Work out the finished part from the listing and answer in its coordinate system (mm). Face numbers are marked on the shaded views. A direction names the side the tool comes from. Round coordinates to 2 decimals unless told otherwise and drop trailing zeros. Order: outer loops, then holes, each group sorted by start corner. A loop starts at its lowest first (then second) coordinate and runs counter-clockwise, first axis right, second up. Notation, with made-up numbers: (39.5, -14.5) -> (93.5, -14.5) arc R30 cw to (93.5, 20.5) -> close; hole circle Ø6 at (-39.5, 13.25). An arc over 180 degrees is marked (long way). Use a Markdown table: item, result. Add a question column.
Item 1: For a pull along Y with two mould halves and no side action, classify the marked faces 1, 2 and 3 as +Y half, -Y half, draft (parallel to the pull), parting line (faces both ways), or undercut.
Item 2: A cutting plane is placed at C-C, the plane y = 49. Determine the outline of the cut face in (x, z), plus the area to 3 significant figures.
Item 3: A cutting plane is placed at B-B, the plane z = 6.25. Determine the outline of the cut face in (x, y).
Item 4: A tool of negligible diameter and unlimited length cuts with its end or side. For the marked faces 4 and 5, from which of +Z, -Z, +X, -X, +Y, -Y can it reach the whole face along a straight path? Write none if from no direction.
Item 5: A cutting plane is placed at A-A, the plane x = -25. Determine the outline of the cut face in (y, z).
Item 6: A cutting plane is placed at D-D, the plane y = -12. Determine the outline of the cut face in (x, z).
Item 7: Flat-ended cylindrical pins translate along their axes: P1, Ø3.5, axis at y = 11.5, z = 3, coming from the +X side; P2, Ø2, axis at x = 7, z = 4, coming from the -Y side; P3, Ø2, axis at x = 18.5, y = 28.5, coming from the +Z side; P4, Ø6, axis at x = 27.5, y = 39.5, coming from the +Z side. Find the tip coordinate at first contact, or state that the pin passes through.
Item 8: Find the intervals of material crossed by L1, parallel to Y at x = 7, z = 8.75; L2, parallel to Y at x = 26, z = 3.75; L3, parallel to Y at x = 25, z = 1.8, in increasing order. Write a range as [from, to].
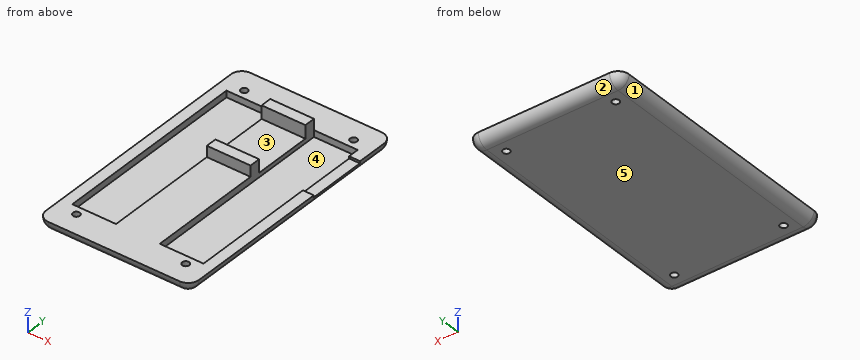
from build123d import *

# Parameters (mm, degrees)
SKETCH_1_W          = 70
SKETCH_1_H          = 118
EXTRUDE_1_DEPTH     = 40
SKETCH_2_W          = 64
SKETCH_2_H          = 112
CUT_EXTRUDE_1_DEPTH = 35
SKETCH_3_R          = 1.6
CUT_EXTRUDE_2_DEPTH = 78.012985918
FILLET_1_R          = 5
FILLET_2_R          = 5
SKETCH_4_W          = 80
SKETCH_4_H          = 120
CUT_EXTRUDE_3_DEPTH = 35
SKETCH_5_W          = 60
SKETCH_5_H          = 27
CUT_EXTRUDE_4_DEPTH = 1
SKETCH_6_W          = 20
SKETCH_6_H          = 90
CUT_EXTRUDE_5_DEPTH = 3
SKETCH_7_W          = 20
SKETCH_7_H          = 90
CUT_EXTRUDE_6_DEPTH = 3
SKETCH_8_W          = 20
SKETCH_8_H          = 5
EXTRUDE_2_DEPTH     = 5


with BuildPart() as part:
    # ｽｹｯﾁ1 → ﾎﾞｽ - 押し出し1 (new body)
    with BuildSketch(Plane.XY):
        Rectangle(SKETCH_1_W, SKETCH_1_H)
    extrude(amount=EXTRUDE_1_DEPTH)

    # ｽｹｯﾁ2 → ｶｯﾄ - 押し出し1 (cut)
    with BuildSketch(Plane.XY.offset(40)):
        Rectangle(SKETCH_2_W, SKETCH_2_H)
    extrude(amount=-CUT_EXTRUDE_1_DEPTH, mode=Mode.SUBTRACT)

    # ｽｹｯﾁ3 → ｶｯﾄ - 押し出し2 (cut, through all)
    with BuildSketch(Plane.XY.offset(5)):
        with Locations((-25, 49)):
            Circle(SKETCH_3_R)
        with Locations((25, 49)):
            Circle(SKETCH_3_R)
        with Locations((-25, -49)):
            Circle(SKETCH_3_R)
        with Locations((25, -49)):
            Circle(SKETCH_3_R)
    extrude(amount=-CUT_EXTRUDE_2_DEPTH, mode=Mode.SUBTRACT)

    # ﾌｨﾚｯﾄ1
    fillet_1_edges = [part.edges().sort_by_distance(p)[0] for p in [
        (0, -59, 0),
        (-35, 0, 0),
        (0, 59, 0),
        (35, 0, 0),
    ]]
    fillet(fillet_1_edges, radius=FILLET_1_R)

    # ﾌｨﾚｯﾄ2
    # the kernel refuses this fillet: 5 mm, written as the material it takes off along each edge
    with BuildSketch(Plane(origin=(-30, 54, 5), x_dir=(0, 1, 0), z_dir=(-1, 0, 0))) as fillet_2_piece_1_section:
        Polygon((0, 0), (FILLET_2_R, 0), (FILLET_2_R, FILLET_2_R), (0, FILLET_2_R), align=None)
    fillet_2_piece_1 = extrude(amount=FILLET_2_R, mode=Mode.PRIVATE)
    fillet_2_piece_1 = fillet_2_piece_1 - Plane(origin=(-30, 54, 5), x_dir=(0, -0.7071067811865475, 0.7071067811865475), z_dir=(-1, 0, 0)) * Sphere(FILLET_2_R, mode=Mode.PRIVATE)
    add(fillet_2_piece_1, mode=Mode.SUBTRACT)
    with BuildSketch(Plane(origin=(30, 54, 5), x_dir=(0, 1, 0), z_dir=(1, 0, 0))) as fillet_2_piece_2_section:
        Polygon((0, 0), (FILLET_2_R, 0), (FILLET_2_R, -FILLET_2_R), (0, -FILLET_2_R), align=None)
    fillet_2_piece_2 = extrude(amount=FILLET_2_R, mode=Mode.PRIVATE)
    fillet_2_piece_2 = fillet_2_piece_2 - Plane(origin=(30, 54, 5), x_dir=(0, -0.7071067811865475, 0.7071067811865475), z_dir=(1, 0, 0)) * Sphere(FILLET_2_R, mode=Mode.PRIVATE)
    add(fillet_2_piece_2, mode=Mode.SUBTRACT)
    with BuildSketch(Plane(origin=(-30, -54, 5), x_dir=(-1, 0, 0), z_dir=(0, -1, 0))) as fillet_2_piece_3_section:
        Polygon((0, 0), (FILLET_2_R, 0), (FILLET_2_R, FILLET_2_R), (0, FILLET_2_R), align=None)
    fillet_2_piece_3 = extrude(amount=FILLET_2_R, mode=Mode.PRIVATE)
    fillet_2_piece_3 = fillet_2_piece_3 - Plane(origin=(-30, -54, 5), x_dir=(0.7071067811865475, 0, 0.7071067811865475), z_dir=(0, -1, 0)) * Sphere(FILLET_2_R, mode=Mode.PRIVATE)
    add(fillet_2_piece_3, mode=Mode.SUBTRACT)
    with BuildSketch(Plane(origin=(30, -54, 5), x_dir=(1, 0, 0), z_dir=(0, -1, 0))) as fillet_2_piece_4_section:
        Polygon((0, 0), (FILLET_2_R, 0), (FILLET_2_R, -FILLET_2_R), (0, -FILLET_2_R), align=None)
    fillet_2_piece_4 = extrude(amount=FILLET_2_R, mode=Mode.PRIVATE)
    fillet_2_piece_4 = fillet_2_piece_4 - Plane(origin=(30, -54, 5), x_dir=(-0.7071067811865475, 0, 0.7071067811865475), z_dir=(0, -1, 0)) * Sphere(FILLET_2_R, mode=Mode.PRIVATE)
    add(fillet_2_piece_4, mode=Mode.SUBTRACT)
    with BuildSketch(Plane(origin=(35, -59, 5), x_dir=(-1, 0, 0), z_dir=(0, 0, 1)), Plane(origin=(35, 59, 5), x_dir=(0, -1, 0), z_dir=(0, 0, 1))) as fillet_2_piece_5:
        with BuildLine():
            CenterArc((FILLET_2_R, -FILLET_2_R), FILLET_2_R, 90, 90)
            Line((0, -FILLET_2_R), (0, 0))
            Line((0, 0), (FILLET_2_R, 0))
        make_face()
    extrude(amount=47.5, mode=Mode.SUBTRACT)
    with BuildSketch(Plane(origin=(-35, -59, 5), x_dir=(1, 0, 0), z_dir=(0, 0, 1)), Plane(origin=(-35, 59, 5), x_dir=(0, -1, 0), z_dir=(0, 0, 1))) as fillet_2_piece_6:
        with BuildLine():
            CenterArc((FILLET_2_R, FILLET_2_R), FILLET_2_R, 180, 90)
            Line((0, FILLET_2_R), (0, 0))
            Line((0, 0), (FILLET_2_R, 0))
        make_face()
    extrude(amount=47.5, mode=Mode.SUBTRACT)

    # ｽｹｯﾁ4 → ｶｯﾄ - 押し出し3 (cut)
    with BuildSketch(Plane.XY.offset(40)):
        Rectangle(SKETCH_4_W, SKETCH_4_H)
    extrude(amount=-CUT_EXTRUDE_3_DEPTH, mode=Mode.SUBTRACT)

    # ｽｹｯﾁ5 → ｶｯﾄ - 押し出し4 (cut)
    with BuildSketch(Plane.XY.offset(5)):
        with Locations((5, 26.5)):
            Rectangle(SKETCH_5_W, SKETCH_5_H)
    extrude(amount=-CUT_EXTRUDE_4_DEPTH, mode=Mode.SUBTRACT)

    # ｽｹｯﾁ6 → ｶｯﾄ - 押し出し5 (cut)
    with BuildSketch(Plane.XY.offset(5)):
        with Locations((-20, 0)):
            Rectangle(SKETCH_6_W, SKETCH_6_H)
    extrude(amount=-CUT_EXTRUDE_5_DEPTH, mode=Mode.SUBTRACT)

    # ｽｹｯﾁ7 → ｶｯﾄ - 押し出し6 (cut)
    with BuildSketch(Plane.XY.offset(5)):
        with Locations((20, 0)):
            Rectangle(SKETCH_7_W, SKETCH_7_H)
    extrude(amount=-CUT_EXTRUDE_6_DEPTH, mode=Mode.SUBTRACT)

    # ｽｹｯﾁ8 → ﾎﾞｽ - 押し出し2 (add)
    with BuildSketch(Plane.XY.offset(5)):
        with Locations((0, 10.5)):
            Rectangle(SKETCH_8_W, SKETCH_8_H)
        with Locations((0, 42.5)):
            Rectangle(SKETCH_8_W, SKETCH_8_H)
    extrude(amount=EXTRUDE_2_DEPTH)


solid = part.part
Reported:
| question | item | result |
|---|---|---|
| 1 | face 1 | draft |
| 1 | face 2 | +Y half |
| 1 | face 3 | undercut |
| 2 | outline | (-35, 5) arc R5 ccw to (-30, 0) -> (-26.6, 0) -> (-26.6, 5) -> close; (-23.4, 0) -> (23.4, 0) -> (23.4, 5) -> (-23.4, 5) -> close; (26.6, 0) -> (30, 0) arc R5 ccw to (35, 5) -> (26.6, 5) -> close |
| 2 | area | 307 mm² |
| 3 | outline | (-10, 8) -> (10, 8) -> (10, 13) -> (-10, 13) -> close; (-10, 40) -> (10, 40) -> (10, 45) -> (-10, 45) -> close |
| 4 | face 4 | +Z |
| 4 | face 5 | -Z, +X, -X, +Y, -Y |
| 5 | outline | (-59, 5) arc R5 ccw to (-54, 0) -> (-50.6, 0) -> (-50.6, 5) -> close; (-47.4, 0) -> (47.4, 0) -> (47.4, 5) -> (45, 5) -> (45, 2) -> (-45, 2) -> (-45, 5) -> (-47.4, 5) -> close; (50.6, 0) -> (54, 0) arc R5 ccw to (59, 5) -> (50.6, 5) -> close |
| 6 | outline | (-35, 5) arc R5 ccw to (-30, 0) -> (30, 0) arc R5 ccw to (35, 5) -> (30, 5) -> (30, 2) -> (10, 2) -> (10, 5) -> (-10, 5) -> (-10, 2) -> (-30, 2) -> (-30, 5) -> close |
| 7 | P1 | x = 34.99 |
| 7 | P2 | y = -59 |
| 7 | P3 | z = 2 |
| 7 | P4 | z = 5 |
| 8 | L1 | [8, 13], [40, 45] |
| 8 | L2 | [-58.84, -50.25], [-47.75, -45], [45, 47.75], [50.25, 58.84] |
| 8 | L3 | [-57.84, -50.6], [-47.4, 47.4], [50.6, 57.84] |
